Drawing for the job (mm, zero at the part's lowest x, y, z). Coordinates: 2 decimals unless noted, no trailing zeros. Write each loop counter-clockwise with the first axis right and the second up, starting at its lowest first coordinate (ties: lowest second). Pieces come first, ordered by that corner, then holes.
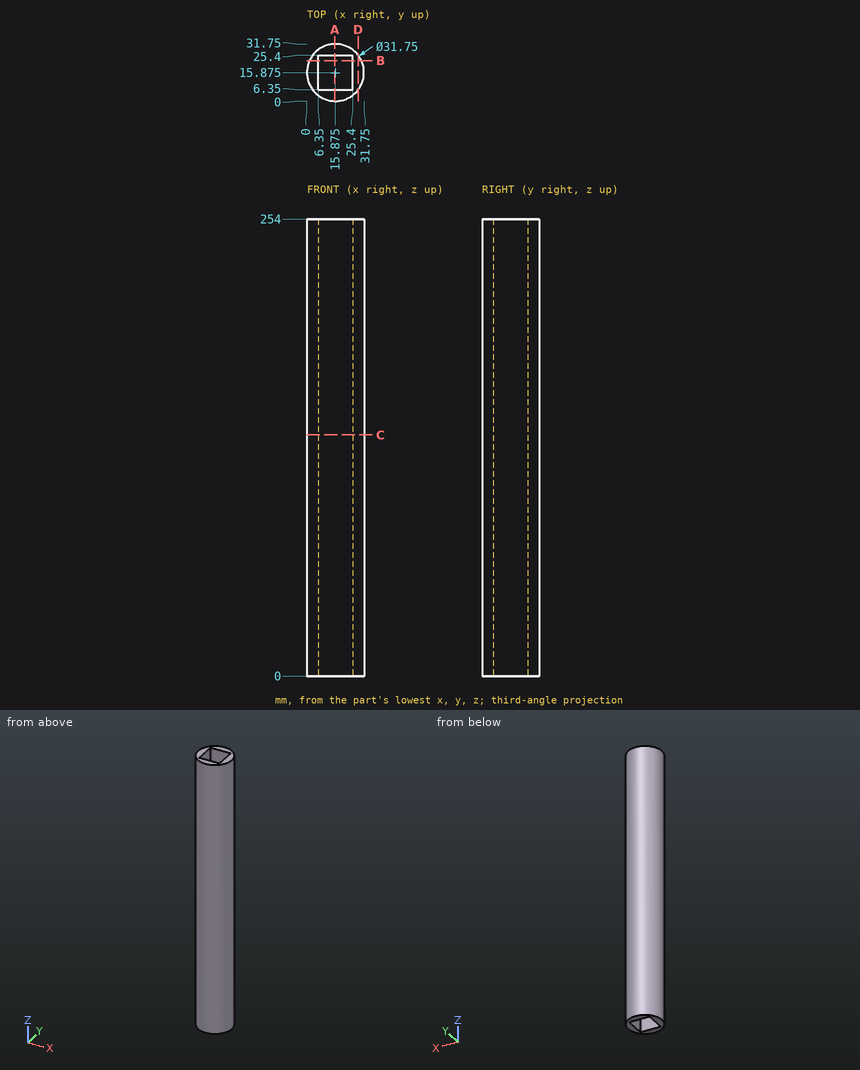
Item 1: Flat gauge pins, fed straight in: pin 1 Ø3 at (x, z) = (9.5, 121) entering from -Y; pin 2 Ø8 at (x, y) = (17.5, 17.5) entering from +Z; pin 3 Ø5 at (y, z) = (25.5, 165) entering from +X; pin 4 Ø8 at (x, z) = (26.5, 116.5) entering from +Y. Where does each tip first touch, or does it go through?
Item 2: Wall check: line 1 along X through (y, z) = (16, 218.5); line 2 along Y through (x, z) = (16.5, 162.5); line 3 along Y through (x, z) = (20, 172). Give the ranges that are in metal, low to high.
Item 3: Saw through at D-D, the plane x = 28.5. Write the cut outline in (y, z), and give its area (3 significant figures).
Item 4: Saw through at C-C, the plane z = 134. Write the cut outline in (x, y) (3 decimals), and give its area (3 significant figures).
Item 5: Saw through at A-A, the plane x = 15.5. Write the cut outline in (y, z), and give its area (3 significant figures).
Item 6: Saw through at B-B, the plane y = 22.5. Write the cut outline in (x, z).
Working result:
1. pin 1: stops at y = 0.77
1. pin 2: passes through
1. pin 3: stops at x = 30.06
1. pin 4: stops at y = 30.3
2. line 1: x = 0 to 6.35, 25.4 to 31.75
2. line 2: y = 0.01 to 6.35, 25.4 to 31.74
2. line 3: y = 0.55 to 6.35, 25.4 to 31.2
3. outline: (6.25, 0) - (25.5, 0) - (25.5, 254) - (6.25, 254) - close
3. area: 4,890 mm2
4. outline: circle Ø31.75 at (15.875, 15.875); hole (6.35, 6.35) - (25.4, 6.35) - (25.4, 25.4) - (6.35, 25.4) - close
4. area: 429 mm2
5. outline: (0, 0) - (6.35, 0) - (6.35, 254) - (0, 254) - close; (25.4, 0) - (31.75, 0) - (31.75, 254) - (25.4, 254) - close
5. area: 3,220 mm2
6. outline: (1.45, 0) - (6.35, 0) - (6.35, 254) - (1.45, 254) - close; (25.4, 0) - (30.3, 0) - (30.3, 254) - (25.4, 254) - close
